from build123d import *

# Parameters (mm, degrees)
SKETCH4_W               = 106
SKETCH4_H               = 25.5
BOSS_EXTRUDE2_DEPTH     = 13
CUT_EXTRUDE3_DEPTH      = 101.130030155
CUT_EXTRUDE3_DEPTH_BACK = 8.3
SKETCH25_W              = 106
SKETCH25_H              = 8.1
M3X0_5_TAPPED_HOLE1_D   = 2.5


with BuildPart() as part:
    # Sketch4 → Boss-Extrude2 (new body)
    with BuildSketch(Plane.XY):
        with Locations((-36.891047602, -29.4)):
            Rectangle(SKETCH4_W, SKETCH4_H)
    extrude(amount=-BOSS_EXTRUDE2_DEPTH)

    # Sketch25 → Cut-Extrude3 (cut, two sides: drawn at the far end of the back side and taken through both)
    with BuildSketch(Plane.XY.offset(-CUT_EXTRUDE3_DEPTH_BACK)):
        with Locations((-36.891047602, -24.98)):
            Rectangle(SKETCH25_W, SKETCH25_H)
    extrude(amount=CUT_EXTRUDE3_DEPTH + CUT_EXTRUDE3_DEPTH_BACK, mode=Mode.SUBTRACT)

    # M3x0.5 Tapped Hole1 (through all)
    with Locations(Plane(origin=(-74.390985602, -16.65, -4.15), x_dir=(0, 0, 1), z_dir=(0, 1, 0))):
        with Locations((0, 0), (0, 25), (-0.055677319, 74.999938), (0, 50)):
            Hole(M3X0_5_TAPPED_HOLE1_D / 2)


solid = part.part
Geometry check sheet. Reference: the model listing, model coordinates, mm. A direction names the side the tool comes from. Give positions to 0.01 mm unless a question says otherwise; leave off trailing zeros. Write each loop counter-clockwise with the first axis right and the second up, starting at its lowest first coordinate (ties: lowest second). Pieces come first, ordered by that corner, then holes.
1) Cross-section at C-C (y = -22.5). Record the boundary of the cut face in (x, z).
Values follow:
outline: (-89.89, -13) - (16.11, -13) - (16.11, -8.3) - (-89.89, -8.3) - close
2) Release check for a two-part mould opening along Z. For faces 1 (the face through (-25.61, -35.68, -3.88)), 2 (the face through (-38, -19, 0)), 3 (the face through (-38, -16.65, -6)), 4 (the face through (-38, -29, -13)) record: released by +Z, released by -Z, zero draft, split by the parting line, or undercut.
Values follow:
face 1: undercut
face 2: released by +Z
face 3: zero draft
face 4: released by -Z
3) Thickness scan on line 1 (X direction, y = -19.95, z = -4.15); line 2 (Y direction, x = -8.5, z = -2); line 3 (Z direction, x = -41, y = -25.5). Record the ranges inside material, lowest first.
Values follow:
line 1: x = -89.89 to -75.64, -73.14 to -50.64, -48.14 to -25.64, -23.14 to -0.64, 1.86 to 16.11
line 2: y = -42.15 to -29.03, -20.93 to -16.65
line 3: z = -13 to -8.3
4) Go/stop test with flat-tipped pins: pin 1 Ø2 at (x, z) = (-49.39, -4.15) entering from -Y; pin 2 Ø2 at (x, y) = (-72, -30) entering from +Z. Record where each tip stops, or that it passes through.
Values follow:
pin 1: passes through
pin 2: stops at z = 0
5) Set-up check for faces 5 (the face through (-48.15, -18.82, -3.99)), 6 (the face through (-38, -20.93, -4)): record each of +Z, -Z, +X, -X, +Y, -Y from which the full face is reachable in a straight line by a thin tool's end or side.
Values follow:
face 5: +Y, -Y
face 6: +Z, +X, -X
6) Cross-section at B-B (x = -55). Record the boundary of the cut face in (y, z), plus the area to 3 significant figures.
Values follow:
outline: (-42.15, -13) - (-16.65, -13) - (-16.65, 0) - (-20.93, 0) - (-20.93, -8.3) - (-29.03, -8.3) - (-29.03, 0) - (-42.15, 0) - close
area: 264 mm2
7) Cross-section at A-A (z = -1.5). Record the boundary of the cut face in (x, y), plus the area to 3 significant figures.
Values follow:
outline: (-89.89, -42.15) - (16.11, -42.15) - (16.11, -29.03) - (-89.89, -29.03) - close; (-89.89, -20.93) - (16.11, -20.93) - (16.11, -16.65) - (-89.89, -16.65) - close
area: 1,840 mm2
